from build123d import *

# Parameters (mm, degrees)
SKETCH1_W           = 165
SKETCH1_H           = 50
BOSS_EXTRUDE1_DEPTH = 2.5
FILLET1_R           = 25
SKETCH2_R           = 2.5
CUT_EXTRUDE1_DEPTH  = 2.5
SKETCH3_R           = 2.5
CUT_EXTRUDE2_DEPTH  = 2.5
SKETCH4_R           = 2.25
BOSS_EXTRUDE2_DEPTH = 8


with BuildPart() as part:
    # Sketch1 → Boss-Extrude1 (new body)
    with BuildSketch(Plane.XY):
        Rectangle(SKETCH1_W, SKETCH1_H)
    extrude(amount=BOSS_EXTRUDE1_DEPTH)

    # Fillet1
    fillet1_edges = [part.edges().sort_by_distance(p)[0] for p in [
        (-82.5, -25, 1.25),
        (-82.5, 25, 1.25),
        (82.5, -25, 1.25),
        (82.5, 25, 1.25),
    ]]
    fillet(fillet1_edges, radius=FILLET1_R - 0.0001)  # a hair under: the kernel refuses the full size

    # Sketch2 → Cut-Extrude1 (cut)
    with BuildSketch(Plane.XY.offset(2.5)):
        with Locations((-5, 20)):
            Circle(SKETCH2_R)
        with Locations((5, 20)):
            Circle(SKETCH2_R)
    cut_extrude1 = extrude(amount=-CUT_EXTRUDE1_DEPTH, mode=Mode.SUBTRACT)

    # Mirror1: Cut-Extrude1 across plane
    add(cut_extrude1.mirror(Plane.ZX), mode=Mode.SUBTRACT)

    # Sketch3 → Cut-Extrude2 (cut)
    with BuildSketch(Plane(origin=(0, 0, 0), x_dir=(-1, 0, 0), z_dir=(0, 0, -1))):
        with Locations((-57.5, 0)):
            Circle(SKETCH3_R)
    extrude(amount=-CUT_EXTRUDE2_DEPTH, mode=Mode.SUBTRACT)

    # Sketch4 → Boss-Extrude2 (add)
    with BuildSketch(Plane.XY.offset(2.5)):
        with Locations(Location((-57.5, 0, 0), (0, 0, 180))):
            Circle(SKETCH4_R)
    extrude(amount=BOSS_EXTRUDE2_DEPTH)


solid = part.part
Geometry check sheet. Reference: the model listing, model coordinates, mm. Give positions to 0.01 mm unless a question says otherwise; leave off trailing zeros. Order: outer loops, then holes, each group sorted by start corner. A loop starts at its lowest first (then second) coordinate and runs counter-clockwise, first axis right, second up.
1) Cross-section at B-B (z = 4.75). Record the boundary of the cut face in (x, y).
Results are:
outline: circle Ø4.5 at (-57.5, 0)
2) Cross-section at D-D (x = -47.5). Record the boundary of the cut face in (y, z).
Results are:
outline: (-25, 0) - (25, 0) - (25, 2.5) - (-25, 2.5) - close
3) Material ranges on probe 1 along Y at (x, z) = (5, 1.3); probe 2 along Y at (x, z) = (57.5, 1.55); probe 3 along X at (y, z) = (-20, 1.25), recorded low to high.
Results are:
probe 1: y = -25 to -22.5, -17.5 to 17.5, 22.5 to 25
probe 2: y = -25 to -2.5, 2.5 to 25
probe 3: x = -72.5 to -7.5, -2.5 to 2.5, 7.5 to 72.5
4) Gauge pin test, flat ends, axial feed: pin 1 (3 mm diameter, centred on x = -59.5, z = 6, fed in from +Y); pin 2 (1 mm diameter, centred on y = -1.5, z = 1.5, fed in from -X); pin 3 (3 mm diameter, centred on x = 48, z = 3.5, fed in from +Y); pin 4 (6 mm diameter, centred on x = -3.5, z = 7.5, fed in from +Y). Record the tip position at first contact, or that the pin passes through.
Results are:
pin 1: stops at y = 2.19
pin 2: stops at x = -82.48
pin 3: stops at y = 25
pin 4: passes through
5) Cross-section at C-C (y = 12.5). Record the boundary of the cut face in (x, z), then the cut area to 3 significant figures.
Results are:
outline: (-79.15, 0) - (79.15, 0) - (79.15, 2.5) - (-79.15, 2.5) - close
area: 396 mm2
6) Cross-section at A-A (x = -5). Record the boundary of the cut face in (y, z).
Results are:
outline: (-25, 0) - (-22.5, 0) - (-22.5, 2.5) - (-25, 2.5) - close; (-17.5, 0) - (17.5, 0) - (17.5, 2.5) - (-17.5, 2.5) - close; (22.5, 0) - (25, 0) - (25, 2.5) - (22.5, 2.5) - close
7) Draft check along X on faces 1 (the cylindrical face through (6.34, -22.11, 1.27)), 2 (the flat face through (-1, 0, 0)), 3 (the cylindrical face through (-55.252, -0.099, 6.444)). Enter one of: released by +X, released by -X, zero draft, split by the parting line, or undercut.
Results are:
face 1: undercut
face 2: zero draft
face 3: split by the parting line
